Geometry check sheet. Reference: the model listing, model coordinates, mm. A direction names the side the tool comes from. Give positions to 0.01 mm unless a question says otherwise; leave off trailing zeros. Write each loop counter-clockwise with the first axis right and the second up, starting at its lowest first coordinate (ties: lowest second). Pieces come first, ordered by that corner, then holes. Notation, with made-up numbers: (83.25, 3) -> (115.25, 3) arc R19 ccw to (115.25, 27) -> close; hole circle Ø9 at (26.25, 76). An arc over 180 degrees is marked (long way). One line per item, written item: value.
from build123d import *

# Parameters (mm, degrees)
SKETCH1_W                       = 300
SKETCH1_H                       = 220
BOSS_EXTRUDE1_DEPTH             = 120
SKETCH3_OUTSIDE_W               = 380.18
SKETCH3_OUTSIDE_H               = 300.18
SKETCH3_OUTSIDE_W_2             = 297
SKETCH3_OUTSIDE_H_2             = 217
CUT_EXTRUDE3_DEPTH              = 30
SKETCH4_R                       = 25
CUT_EXTRUDE4_DEPTH              = 15
FILLET1_R                       = 3
FILLET2_R                       = 5
FILLET3_R                       = 10
F_6_0MM_DOWEL_HOLE1_D           = 6
F_6_0MM_DOWEL_HOLE1_DEPTH       = 30
F_6_0MM_DOWEL_HOLE1_CSINK_D     = 6.05
F_6_0MM_DOWEL_HOLE1_CSINK_ANGLE = 90
F_6_0MM_DOWEL_HOLE1_TIP         = 1.802581857
SKETCH10_R                      = 55
SKETCH10_R_2                    = 45
CUT_EXTRUDE5_DEPTH              = 1
SKETCH11_R                      = 9
CUT_EXTRUDE6_DEPTH              = 30


with BuildPart() as part:
    # Sketch1 → Boss-Extrude1 (new body)
    with BuildSketch(Plane(origin=(0, 0, 0), x_dir=(1, 0, 0), z_dir=(0, 1, 0))):
        Rectangle(SKETCH1_W, SKETCH1_H)
    extrude(amount=BOSS_EXTRUDE1_DEPTH)

    # Sketch3 outside → Cut-Extrude3 (cut)
    with BuildSketch(Plane(origin=(0, 120, 0), x_dir=(1, 0, 0), z_dir=(0, 1, 0))):
        Rectangle(SKETCH3_OUTSIDE_W, SKETCH3_OUTSIDE_H)
        Rectangle(SKETCH3_OUTSIDE_W_2, SKETCH3_OUTSIDE_H_2, mode=Mode.SUBTRACT)
    extrude(amount=-CUT_EXTRUDE3_DEPTH, mode=Mode.SUBTRACT)

    # Sketch4 → Cut-Extrude4 (cut)
    with BuildSketch(Plane(origin=(0, 120, 0), x_dir=(1, 0, 0), z_dir=(0, 1, 0))):
        with Locations((-148.5, -108.5)):
            Circle(SKETCH4_R)
        with Locations((-148.5, 108.5)):
            Circle(SKETCH4_R)
        with Locations((148.5, 108.5)):
            Circle(SKETCH4_R)
        with Locations((148.5, -108.5)):
            Circle(SKETCH4_R)
    extrude(amount=-CUT_EXTRUDE4_DEPTH, mode=Mode.SUBTRACT)

    # Fillet1
    fillet1_edges = [part.edges().sort_by_distance(p)[0] for p in [
        (148.5, 112.5, 83.5),
        (123.5, 112.5, 108.5),
        (123.5, 112.5, -108.5),
        (148.5, 112.5, -83.5),
        (-123.5, 112.5, -108.5),
        (-148.5, 112.5, -83.5),
        (-123.5, 112.5, 108.5),
        (-148.5, 112.5, 83.5),
    ]]
    fillet(fillet1_edges, radius=FILLET1_R)

    # Fillet2
    fillet2_edges = [part.edges().sort_by_distance(p)[0] for p in [
        (148.5, 97.5, -108.5),
        (148.5, 97.5, 108.5),
        (-148.5, 97.5, 108.5),
        (-148.5, 97.5, -108.5),
    ]]
    fillet(fillet2_edges, radius=FILLET2_R)

    # Fillet3
    fillet3_edges = [part.edges().sort_by_distance(p)[0] for p in [
        (-150, 45, -110),
        (150, 45, -110),
        (150, 45, 110),
        (-150, 45, 110),
    ]]
    fillet(fillet3_edges, radius=FILLET3_R)

    # Ø6.0mm Dowel Hole1
    with Locations(Plane(origin=(0, 105, 0), x_dir=(1, 0, 0), z_dir=(0, 1, 0))):
        with Locations((-137.151874048, 97.743982636), (-137.151874048, -98.364579351), (139.323962551, -98.364579351), (139.323962551, 97.743982636)):
            CounterSinkHole(F_6_0MM_DOWEL_HOLE1_D / 2, F_6_0MM_DOWEL_HOLE1_CSINK_D / 2, depth=F_6_0MM_DOWEL_HOLE1_DEPTH, counter_sink_angle=F_6_0MM_DOWEL_HOLE1_CSINK_ANGLE)
            with Locations((0, 0, -(F_6_0MM_DOWEL_HOLE1_DEPTH + F_6_0MM_DOWEL_HOLE1_TIP / 2))):  # 118° drill point
                Cone(0, F_6_0MM_DOWEL_HOLE1_D / 2, F_6_0MM_DOWEL_HOLE1_TIP, mode=Mode.SUBTRACT)

    # Sketch10 → Cut-Extrude5 (cut)
    with BuildSketch(Plane(origin=(0, 120, 0), x_dir=(1, 0, 0), z_dir=(0, 1, 0))):
        with Locations(Location((-78.5, -38.5, 0), (0, 0, 270))):
            Circle(SKETCH10_R)
        with Locations(Location((88.5, 48.5, 0), (0, 0, 270))):
            Circle(SKETCH10_R_2)
    extrude(amount=-CUT_EXTRUDE5_DEPTH, mode=Mode.SUBTRACT)

    # Sketch11 → Cut-Extrude6 (cut)
    with BuildSketch(Plane.XZ):
        with Locations(Location((120, 0, 0), (0, 0, 270))):
            Circle(SKETCH11_R)
        with Locations(Location((60, 0, 0), (0, 0, 270))):
            Circle(SKETCH11_R)
        with Locations(Location((-125, -75, 0), (0, 0, 270))):
            Circle(SKETCH11_R)
    extrude(amount=-CUT_EXTRUDE6_DEPTH, mode=Mode.SUBTRACT)


solid = part.part
1) Scan lines: probe 1 along X at (y, z) = (7.5, 0); probe 2 along X at (y, z) = (93.5, -98); probe 3 along X at (y, z) = (15, -75). Record each from-to range of solid material in increasing order.
Verdict:
probe 1: -150 to 51, 69 to 111, 129 to 150
probe 2: -148.5 to -140.14, -134.16 to 136.33, 142.31 to 148.5
probe 3: -150 to -134, -116 to 150
2) Mould release check, pull along Z, two halves, no side actions. Record for faces 1 (the cylindrical face through (130.655, 112.605, -90.991)), 2 (the conical face through (-136.67, 73.51, 98.56)), 3 (the flat face through (134, 105, 97)): released by +Z, released by -Z, zero draft, split by the parting line, or undercut.
Verdict:
face 1: released by -Z
face 2: undercut
face 3: zero draft
3) Sectioned sample at C-C on z = -75. Record the cut outline in (x, y).
Verdict:
outline: (-150, 0) -> (-134, 0) -> (-134, 30) -> (-116, 30) -> (-116, 0) -> (150, 0) -> (150, 90) -> (148.5, 90) -> (148.5, 120) -> (124.87, 120) -> (124.87, 119) -> (52.13, 119) -> (52.13, 120) -> (-148.5, 120) -> (-148.5, 90) -> (-150, 90) -> close
4) Depth check by flat-ended pin: pin 1 Ø24 at (y, z) = (107.5, 31.5) entering from +X; pin 2 Ø8 at (x, z) = (-58.5, 41) entering from +Y. Enter the tip coordinate at first touch or a pass-through.
Verdict:
pin 1: x = 148.5
pin 2: y = 119
5) Tool access check on faces 4 (the flat face through (-125, 30, -75)), 5 (the flat face through (-141, 105, -98)), 6 (the flat face through (148.5, 105, 1)). Record the directions out of +Z, -Z, +X, -X, +Y, -Y that give a thin tool (end or side, any length) a straight path to the whole face; none if there is none.
Verdict:
face 4: -Y
face 5: -Z, -X, +Y
face 6: +Z, -Z, +X, +Y
6) Sectioned sample at B-B on z = 0. Record the cut outline in (x, y), plus the area to 3 significant figures.
Verdict:
outline: (-150, 0) -> (51, 0) -> (51, 30) -> (69, 30) -> (69, 0) -> (111, 0) -> (111, 30) -> (129, 30) -> (129, 0) -> (150, 0) -> (150, 90) -> (148.5, 90) -> (148.5, 120) -> (-39.22, 120) -> (-39.22, 119) -> (-117.78, 119) -> (-117.78, 120) -> (-148.5, 120) -> (-148.5, 90) -> (-150, 90) -> close
area: 34,800 mm^2
7) Sectioned sample at A-A on y = 94.5. Record the cut outline in (x, z), plus the area to 3 significant figures.
Verdict:
outline: (-148.5, -103.5) arc R5 ccw to (-143.5, -108.5) -> (143.5, -108.5) arc R5 ccw to (148.5, -103.5) -> (148.5, 103.5) arc R5 ccw to (143.5, 108.5) -> (-143.5, 108.5) arc R5 ccw to (-148.5, 103.5) -> close; hole circle Ø6 at (-137.15, -97.74); hole circle Ø6 at (-137.15, 98.36); hole circle Ø6 at (139.32, -97.74); hole circle Ø6 at (139.32, 98.36)
area: 64,300 mm^2
